Build history of the part. All positions in model axes, mm. Round coordinates to 2 decimals unless told otherwise and drop trailing zeros. Write each loop counter-clockwise with the first axis right and the second up, starting at its lowest first coordinate (ties: lowest second). Pieces come first, ordered by that corner, then holes. Notation, with made-up numbers: M -15,72.5 L 1,72.5 A7 ccw 1,80.5 Z; hole C 37,85 d4. An arc over 180 degrees is marked long. One line per item, written item: value. Start each with the question number.
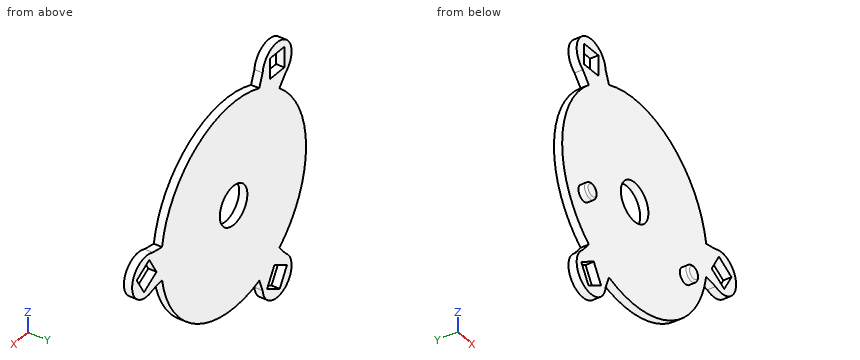
```python
from build123d import *

# Parameters (mm, degrees)
SKETCH1_R           = 25
SKETCH1_W           = 5
SKETCH1_H           = 5
BOSS_EXTRUDE1_DEPTH = 2
CUT_EXTRUDE1_REACH  = 4
SKETCH2_R           = 4.75
SKETCH3_R           = 1.9
BOSS_EXTRUDE2_DEPTH = 2
FILLET1_R           = 0.5


with BuildPart() as part:
    # Sketch1 → Boss-Extrude1 (new body)
    with BuildSketch(Plane(origin=(0, 0, 0), x_dir=(1, 0, 0), z_dir=(0, 1, 0))):
        Circle(SKETCH1_R)
        with BuildLine():
            Line((0, 0), (-17.886625066, -21.898189918))
            ThreePointArc((-17.886625066, -21.898189918), (-17.5, -30.310889132), (-10.021076233, -26.439366654))
            Line((-10.021076233, -26.439366654), (0, 0))
        make_face()
        with Locations((-15, -25.980762114)):
            Rectangle(SKETCH1_W, SKETCH1_H, mode=Mode.SUBTRACT)
        with BuildLine():
            Line((0, 0), (27.907701299, -4.541176736))
            ThreePointArc((27.907701299, -4.541176736), (35, 0), (27.907701299, 4.541176736))
            Line((27.907701299, 4.541176736), (0, 0))
        make_face()
        Polygon((29.084936491, -3.415063509), (26.584936491, 0.915063509), (30.915063509, 3.415063509), (33.415063509, -0.915063509), align=None, mode=Mode.SUBTRACT)
        with BuildLine():
            Line((0, 0), (-10.021076233, 26.439366654))
            ThreePointArc((-10.021076233, 26.439366654), (-17.5, 30.310889132), (-17.886625066, 21.898189918))
            Line((-17.886625066, 21.898189918), (0, 0))
        make_face()
        Polygon((-11.584936491, 26.895825623), (-14.084936491, 22.565698604), (-18.415063509, 25.065698604), (-15.915063509, 29.395825623), align=None, mode=Mode.SUBTRACT)
    extrude(amount=BOSS_EXTRUDE1_DEPTH)

    # Sketch2 → Cut-Extrude1 (cut, up to next)
    with BuildSketch(Plane(origin=(0, 0, 0), x_dir=(-1, 0, 0), z_dir=(0, -1, 0)), mode=Mode.PRIVATE) as cut_extrude1_sk1:
        Circle(SKETCH2_R)
    cut_extrude1_tool1 = extrude(cut_extrude1_sk1.sketch, amount=-CUT_EXTRUDE1_REACH, mode=Mode.PRIVATE) & part.part
    add(cut_extrude1_tool1.solids().sort_by_distance((0, 0, 0))[0], mode=Mode.SUBTRACT)

    # Sketch3 → Boss-Extrude2 (add)
    with BuildSketch(Plane(origin=(0, 0, 0), x_dir=(-1, 0, 0), z_dir=(0, -1, 0))):
        with Locations((17.5, 8)):
            Circle(SKETCH3_R)
        with Locations((-17.5, 8)):
            Circle(SKETCH3_R)
    extrude(amount=BOSS_EXTRUDE2_DEPTH)

    # Fillet1
    fillet1_edges = [part.edges().sort_by_distance(p)[0] for p in [
        (-15.6, -2, -8),
        (19.4, -2, -8),
    ]]
    fillet(fillet1_edges, radius=FILLET1_R)


solid = part.part
```
Item 1: Cut at D-D, the plane z = -8. Write the cut outline in (x, y), plus the area to 3 significant figures.
Item 2: Cut at A-A, the plane x = 0. Write the cut outline in (y, z), plus the area to 3 significant figures.
Item 3: Cut at B-B, the plane y = 0.65. Write the cut outline in (x, z), plus the area to 3 significant figures.
Item 4: Drill centre lines: line 1 (Z direction, x = 0, y = 0.5); line 2 (X direction, y = 1.05, z = 0); line 3 (X direction, y = 1.4, z = 3). Where is each one in solid material? Low to high.
Item 5: Drop flat-ended pins along their axis: pin 1 (6 mm diameter, centred on x = -4, z = -5, fed in from -Y); pin 2 (2 mm diameter, centred on y = 1.5, z = 23.5, fed in from +X); pin 3 (8.5 mm diameter, centred on x = 0, z = 0, fed in from +Y); pin 4 (0.6 mm diameter, centred on y = 1, z = 26, fed in from -X). Give the stop position or say it passes through.
Item 6: Cut at C-C, the plane z = 0. Write the cut outline in (x, y), plus the area to 3 significant figures.
Computed values:
1. outline: M -23.69,0 L -19.4,0 L -19.4,-1.5 A0.5 ccw -18.9,-2 L -16.1,-2 A0.5 ccw -15.6,-1.5 L -15.6,0 L 15.6,0 L 15.6,-1.5 A0.5 ccw 16.1,-2 L 18.9,-2 A0.5 ccw 19.4,-1.5 L 19.4,0 L 23.69,0 L 23.69,2 L -23.69,2 Z
1. area: 110 mm2
2. outline: M 0,-25 L 2,-25 L 2,-4.75 L 0,-4.75 Z; M 0,4.75 L 2,4.75 L 2,25 L 0,25 Z
2. area: 81.0 mm2
3. outline: M -17.89,-21.9 A5 ccw long -10.02,-26.44 L -8.86,-23.38 A25 ccw 24.68,-4.02 L 27.91,-4.54 A5 ccw long 27.91,4.54 L 24.68,4.02 A25 ccw -8.86,23.38 L -10.02,26.44 A5 ccw long -17.89,21.9 L -15.82,19.36 A25 ccw -15.82,-19.36 Z; hole M -18.42,-25.07 L -15.92,-29.4 L -11.58,-26.9 L -14.08,-22.57 Z; hole M -17.5,23.48 L -12.5,23.48 L -12.5,28.48 L -17.5,28.48 Z; hole C 0,0 d9.5; hole M 26.58,-0.92 L 30.92,-3.42 L 33.42,0.92 L 29.08,3.42 Z
3. area: 2,070 mm2
4. line 1: z = -25 to -4.75, 4.75 to 25
4. line 2: x = -25 to -4.75, 4.75 to 27.11, 32.89 to 35
4. line 3: x = -24.82 to -3.68, 3.68 to 28.85, 29.8 to 34
5. pin 1: stops at y = 0
5. pin 2: stops at x = 10.9
5. pin 3: passes through
5. pin 4: stops at x = -20
6. outline: M -25,0 L -4.75,0 L -4.75,2 L -25,2 Z; M 4.75,0 L 27.11,0 L 27.11,2 L 4.75,2 Z; M 32.89,0 L 35,0 L 35,2 L 32.89,2 Z
6. area: 89.5 mm2
